Geometry: see drawing. Coordinates: mm, zero at the bounding-box minimum. A direction names the side the tool comes from. Coordinates: 2 decimals unless noted, no trailing zeros. Loops run counter-clockwise (first coordinate to the right, second up) from the corner with the lowest first, then second, coordinate; pieces in that order, holes last. Notation, with made-up numbers: (71, 51.5) - (84, 51.5) arc R20 cw to (84, 74.5) - close; hole circle Ø11 at (75.5, -12.5). An arc over 180 degrees is marked (long way). Answer in a Markdown table with one row per item.
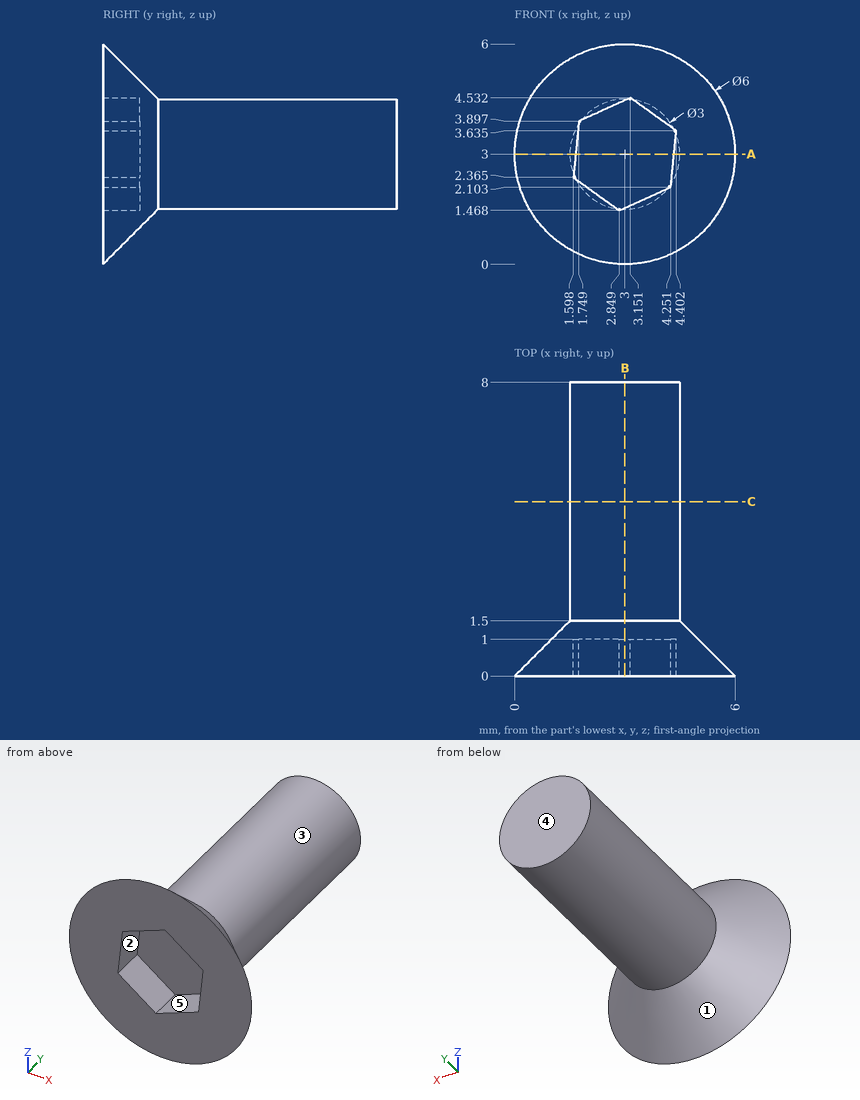
(1) First-contact query: pin 1 Ø1 at (x, z) = (4.5, 5.5) entering from +Y (1 decimal); pin 2 Ø3 at (y, z) = (3.5, 3.5) entering from -X. Flat tips, straight axial feed; report the tip coordinate or a pass-through.
Verdict:
| item | result |
|---|---|
| pin 1 | stops at y = 0.6 |
| pin 2 | stops at x = 1.5 |
(2) Access query for the marked faces 1 and 2. Directions: +Z, -Z, +X, -X, +Y, -Y. A direction counts if a zero-diameter tool reaches every point of the face in a straight line with its end or side. Return the directions, or none.
Verdict:
| item | result |
|---|---|
| face 1 | +Y |
| face 2 | -Y |
(3) Cut plane C-C on y = 4.75. Output: boundary loops of the cut face in (x, z).
Verdict:
| item | result |
|---|---|
| outline | circle Ø3 at (3, 3) |
(4) Cut plane A-A on z = 3. Output: boundary loops of the cut face in (x, y).
Verdict:
| item | result |
|---|---|
| outline | (0, 0) - (1.66, 0) - (1.66, 1) - (4.34, 1) - (4.34, 0) - (6, 0) - (4.5, 1.5) - (4.5, 8) - (1.5, 8) - (1.5, 1.5) - close |
(5) Ray query, probe 1 along Y at (x, z) = (2.1, 2.7); probe 2 along Z at (x, y) = (2.95, 4.25). Return the intervals inside material, ascending.
Verdict:
| item | result |
|---|---|
| probe 1 | y = 1 to 8 |
| probe 2 | z = 1.5 to 4.5 |
(6) Pull-direction query (Z, two-part tool) for the marked faces 3, 4 and 5; classes: pulls with the +Z half, pulls with the -Z half, needs draft (parallel to the pull), parting line crosses it, or undercut.
Verdict:
| item | result |
|---|---|
| face 3 | parting line crosses it |
| face 4 | needs draft |
| face 5 | undercut |
(7) Cut plane B-B on x = 3. Output: boundary loops of the cut face in (y, z).
Verdict:
| item | result |
|---|---|
| outline | (0, 0) - (1.5, 1.5) - (8, 1.5) - (8, 4.5) - (1.5, 4.5) - (0, 6) - (0, 4.46) - (1, 4.46) - (1, 1.54) - (0, 1.54) - close |
